from build123d import *

# Parameters (mm, degrees)
REVOLVE1_ANGLE           = 30
REVOLVE1_OTHER_WAY_ANGLE = 60
REVOLVE2_ANGLE           = 8
REVOLVE2_OTHER_WAY_ANGLE = 8
FILLET1_R                = 5
REVOLVE3_ANGLE           = 7.5
REVOLVE3_OTHER_WAY_ANGLE = 7.5


with BuildPart() as part:
    # Sketch2 → Revolve1 (revolve)
    with BuildSketch(Plane.XY):
        with BuildLine():
            Line((-124.25, 215.20731284), (-122.5, 212.176223927))
            ThreePointArc((-122.5, 212.176223927), (-115.020532883, 216.32216025), (-107.400930963, 220.204541343))
            Line((-107.400930963, 220.204541343), (-109.592786697, 224.698511575))
            ThreePointArc((-109.592786697, 224.698511575), (-126.88459074, 215.40729011), (-143.394109088, 204.788011072))
            Line((-143.394109088, 204.788011072), (-142.533744433, 203.559283006))
            ThreePointArc((-142.533744433, 203.559283006), (-133.518952674, 209.582774285), (-124.25, 215.20731284))
        make_face()
    revolve(axis=Axis((0, 0, 0), (0, 1, 0)), revolution_arc=REVOLVE1_ANGLE)

    # Sketch2 → Revolve1 other way (revolve)
    with BuildSketch(Plane.XY):
        with BuildLine():
            Line((-124.25, 215.20731284), (-122.5, 212.176223927))
            ThreePointArc((-122.5, 212.176223927), (-115.020532883, 216.32216025), (-107.400930963, 220.204541343))
            Line((-107.400930963, 220.204541343), (-109.592786697, 224.698511575))
            ThreePointArc((-109.592786697, 224.698511575), (-126.88459074, 215.40729011), (-143.394109088, 204.788011072))
            Line((-143.394109088, 204.788011072), (-142.533744433, 203.559283006))
            ThreePointArc((-142.533744433, 203.559283006), (-133.518952674, 209.582774285), (-124.25, 215.20731284))
        make_face()
    revolve(axis=Axis((0, 0, 0), (0, -1, 0)), revolution_arc=REVOLVE1_OTHER_WAY_ANGLE)

    # Sketch3 → Revolve2 (revolve)
    with BuildSketch(Plane.XY):
        with BuildLine():
            ThreePointArc((-108.49685883, 222.451526459), (-86.676326862, 231.826366839), (-64.057713663, 239.066642007))
            Line((-64.057713663, 239.066642007), (-64.704761276, 241.481456572))
            ThreePointArc((-64.704761276, 241.481456572), (-87.551845315, 234.168047312), (-109.592786697, 224.698511575))
            Line((-109.592786697, 224.698511575), (-108.49685883, 222.451526459))
        make_face()
    revolve(axis=Axis((0, 0, 0), (0, 1, 0)), revolution_arc=REVOLVE2_ANGLE)

    # Sketch3 → Revolve2 other way (revolve)
    with BuildSketch(Plane.XY):
        with BuildLine():
            ThreePointArc((-108.49685883, 222.451526459), (-86.676326862, 231.826366839), (-64.057713663, 239.066642007))
            Line((-64.057713663, 239.066642007), (-64.704761276, 241.481456572))
            ThreePointArc((-64.704761276, 241.481456572), (-87.551845315, 234.168047312), (-109.592786697, 224.698511575))
            Line((-109.592786697, 224.698511575), (-108.49685883, 222.451526459))
        make_face()
    revolve(axis=Axis((0, 0, 0), (0, -1, 0)), revolution_arc=REVOLVE2_OTHER_WAY_ANGLE)

    # Fillet1
    fillet1_edges = [part.edges().sort_by_distance(p)[0] for p in [
        (-63.754683692, 240.274049289, -8.960136462),
        (-63.754683692, 240.274049289, 8.960136462),
    ]]
    fillet(fillet1_edges, radius=FILLET1_R)

    # Sketch4 → Cut-Revolve1 (revolve, cut)
    with BuildSketch(Plane.XY):
        Polygon((-75.028736809, 245.948635315), (-72.508257021, 237.68635355), (-71.551772701, 237.97813728), (-74.110273038, 246.365052654), align=None)
        Polygon((-74.110273038, 246.365052654), (-71.551772701, 237.97813728), (-68.682319741, 238.853488471), (-71.354881726, 247.614304673), align=None)
        with BuildLine():
            Line((-72.508257021, 237.68635355), (-58.356746094, 191.296864024))
            ThreePointArc((-58.356746094, 191.296864024), (-57.878320073, 191.442158538), (-57.39953231, 191.586256529))
            Line((-57.39953231, 191.586256529), (-71.551772701, 237.97813728))
            Line((-71.551772701, 237.97813728), (-72.508257021, 237.68635355))
        make_face()
    revolve(axis=Axis((0, 0, 0), (-0.2917837304684816, 0.9564843201192044, 0)), mode=Mode.SUBTRACT)

    # Sketch7 → Revolve3 (revolve)
    with BuildSketch(Plane.XY):
        with BuildLine():
            ThreePointArc((-133.400699518, 205.497575091), (-130.717474001, 207.214724358), (-128.012148355, 208.896840267))
            Line((-128.012148355, 208.896840267), (-129.057145485, 210.602120595))
            ThreePointArc((-129.057145485, 210.602120595), (-130.890058266, 209.467879751), (-132.713003262, 208.317687116))
            Line((-132.713003262, 208.317687116), (-133.518952674, 209.582774285))
            ThreePointArc((-133.518952674, 209.582774285), (-134.41391709, 209.009925345), (-135.306423797, 208.433254735))
            Line((-135.306423797, 208.433254735), (-133.400699518, 205.497575091))
        make_face()
    revolve(axis=Axis((0, 0, 0), (0, 1, 0)), revolution_arc=REVOLVE3_ANGLE)

    # Sketch7 → Revolve3 other way (revolve)
    with BuildSketch(Plane.XY):
        with BuildLine():
            ThreePointArc((-133.400699518, 205.497575091), (-130.717474001, 207.214724358), (-128.012148355, 208.896840267))
            Line((-128.012148355, 208.896840267), (-129.057145485, 210.602120595))
            ThreePointArc((-129.057145485, 210.602120595), (-130.890058266, 209.467879751), (-132.713003262, 208.317687116))
            Line((-132.713003262, 208.317687116), (-133.518952674, 209.582774285))
            ThreePointArc((-133.518952674, 209.582774285), (-134.41391709, 209.009925345), (-135.306423797, 208.433254735))
            Line((-135.306423797, 208.433254735), (-133.400699518, 205.497575091))
        make_face()
    revolve(axis=Axis((0, 0, 0), (0, -1, 0)), revolution_arc=REVOLVE3_OTHER_WAY_ANGLE)


solid = part.part
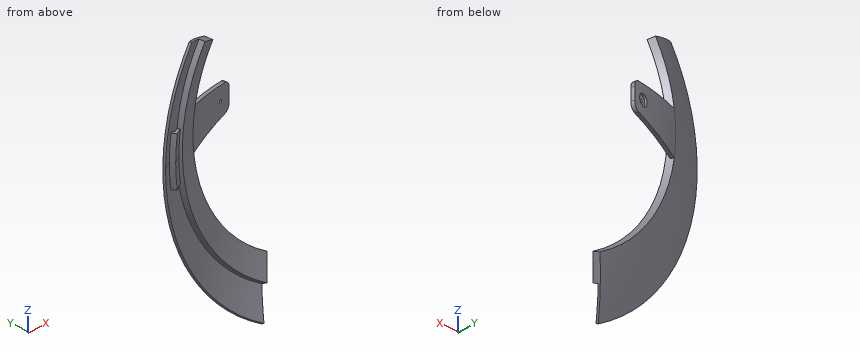
The model under review builds one solid part; all positions refer to its coordinate system, in mm. Round coordinates to 2 decimals unless told otherwise and drop trailing zeros. Loops run counter-clockwise (first coordinate to the right, second up) from the corner with the lowest first, then second, coordinate; pieces in that order, holes last. Notation, with made-up numbers: M 15.25,22.25 L 31.25,22.25 A19 ccw 31.25,55.25 Z; hole C 69,20.25 d8. An arc over 180 degrees is marked long. Answer as a JSON object with one key per item and string values.
Item 1: For line 1 along Z through (x, y) = (-83, 234.5); line 2 along Z through (x, y) = (-92, 210); line 3 along Y through (x, z) = (-136.5, 18), list the stretches that pass through material, from the lowest coordinate up.
Check sheet entries:
{"line 1": "-11.66 to 11.66", "line 2": "-99.68 to -95.86", "line 3": "206.87 to 208.67"}
Item 2: Clearance check with flat-ended pins moving along their axes: P1, Ø5, axis at x = -134, z = 36.5, coming from the +Y side; P2, Ø8, axis at y = 211, z = -18.5, coming from the -X side; P3, Ø3, axis at x = -66, y = 212, coming from the -Z side. State where each tip first meets the part, or that it passes through.
Check sheet entries:
{"P1": "y = 209.52", "P2": "x = -138.98", "P3": "z = -116.18"}
Item 3: We need section A-A, the plane y = 230.5. State the section outline as (x, z) points, and give its area (3 significant figures).
Check sheet entries:
{"outline": "M -95.86,-13.47 L -89.27,-12.55 A90.14 cw -89.27,12.55 L -95.86,13.47 A96.8 ccw Z", "area": "174 mm2"}
